Build history of the part. All positions in model axes, mm. Face numbers are marked on the shaded views. A direction names the side the tool comes from. Give positions to 0.01 mm unless a question says otherwise; leave off trailing zeros. Write each loop counter-clockwise with the first axis right and the second up, starting at its lowest first coordinate (ties: lowest second). Pieces come first, ordered by that corner, then holes. Notation, with made-up numbers: (4, 0) -> (13, 0) arc R18 ccw to (13, 18) -> close; hole circle Ø4 at (89.25, -21). An arc over 180 degrees is marked (long way). Put each result on its own line as item: value.
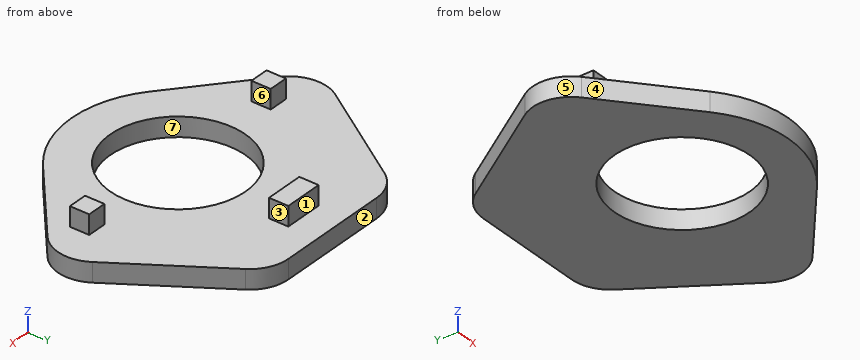
Autodesk Inventor part; units mm, degrees
ref_plane "YZ Plane" through (0, 0, 0) normal (1, 0, 0) x (0, 1, 0)
ref_plane "XZ Plane" through (0, 0, 0) normal (0, 1, 0) x (-1, 0, 0)
ref_plane "XY Plane" through (0, 0, 0) normal (0, 0, 1) x (1, 0, 0)
sketch "Sketch1" plane through (0, 0, 0) normal (0, 0, 1) x (1, 0, 0)
  circle A0 centre (0, 0) radius 7
  circle A1 centre (0, 0) radius 11
  line L0 (-31.215, 0) -> (-15, 0) construction
  line L1 (-11.7494, 0) -> (27.9854, 0) construction
  line L2 (7.0707, -8.4265) -> (18, 0.7443)
  line L3 (18, 0.7443) -> (8, 16)
  line L4 (8, 16) -> (0, 16)
  line L5 (0, -17.2006) -> (0, 31.2913) construction
  line L6 (-7.0707, -8.4265) -> (-18, 0.7443)
  line L7 (-18, 0.7443) -> (-8, 16)
  line L8 (-8, 16) -> (0, 16)
  dimension "d12" = 22
  dimension "d11" = 14
  dimension "d13" = 50
  dimension "d14" = 18
  dimension "d15" = 16
  dimension "d16" = 8
extrude "Extrusion1" add sketch "Sketch1" along normal blind 2
sketch "Sketch2" plane through (0, 0, 2) normal (0, 0, 1) x (1, 0, 0)
  arc A0 (-7.0707, -8.4265) -> (7.0707, -8.4265) centre (0, 0) ccw
  line L0 (7.0707, -8.4265) -> (18, 0.7443)
  line L1 (18, 0.7443) -> (8, 16)
  line L2 (8, 16) -> (-8, 16)
  line L3 (-8, 16) -> (-18, 0.7443)
  line L4 (-18, 0.7443) -> (-7.0707, -8.4265)
  circle A1 centre (0, 0) radius 7
  line L5 (11, -1) -> (13, -1)
  line L6 (13, -1) -> (13, 1)
  line L7 (13, 1) -> (11, 1)
  line L8 (11, 1) -> (11, -1)
  line L9 (11, -1) -> (13, 1) construction
  line L10 (13, -1) -> (11, 1) construction
  line L11 (-2, 13) -> (2, 13)
  line L12 (2, 13) -> (2, 11)
  line L13 (2, 11) -> (-2, 11)
  line L14 (-2, 11) -> (-2, 13)
  line L15 (-2, 13) -> (2, 11) construction
  line L16 (2, 13) -> (-2, 11) construction
  line L17 (0, 16) -> (0, -7) construction
  line L18 (-11, -1) -> (-13, -1)
  line L19 (-13, -1) -> (-13, 1)
  line L20 (-13, 1) -> (-11, 1)
  line L21 (-11, 1) -> (-11, -1)
  line L22 (-11, -1) -> (-13, 1) construction
  line L23 (-13, -1) -> (-11, 1) construction
  point P0 (12, 0)
  point P1 (0, 12)
  point P2 (12, 0)
  point P3 (0, 12)
  point P4 (0, 12)
  point P5 (-12, 0)
  point P6 (-12, 0)
  dimension "d18" = 2
  dimension "d19" = 2
  dimension "d20" = 4
  dimension "d21" = 2
  dimension "d22" = 12
  dimension "d23" = 12
extrude "Extrusion2" add sketch "Sketch2" along normal blind 2 contours L8 L7 L6 L5 | L11 L12 L13 L14 | L18 L19 L20 L21
fillet "Fillet1" radius 4 4 edges at (18, 0.7443, 1) (-18, 0.7443, 1) (-8, 16, 1) (8, 16, 1)
properties part number "lager opvulling voor lijm"
1) Tool access for the marked faces 1, 2 and 3: list every direction of +Z, -Z, +X, -X, +Y, -Y with a clear straight run to the whole face (end or side of a thin tool).
Filled sheet:
face 1: +Z, +X, -X, +Y
face 2: +Z, -Z, +X, -X, +Y
face 3: +Z, +X, +Y, -Y
2) Pin check, flat tips, straight feed: pin 1 (3 mm diameter, centred on x = 4.5, y = 1, fed in from -Z); pin 2 (1.5 mm diameter, centred on x = -5, y = 13, fed in from +Z); pin 3 (1.5 mm diameter, centred on x = 6.5, y = -4, fed in from -Z); pin 4 (1 mm diameter, centred on x = -12.5, z = 3, fed in from +Y). Stop position of each tip, or through.
Filled sheet:
pin 1: through
pin 2: z = 2
pin 3: z = 0
pin 4: y = 1
3) Slice it at B-B (y = -4.5). Write the cut outline in (x, z), plus the area to 3 significant figures.
Filled sheet:
outline: (-11.75, 0) -> (-5.36, 0) -> (-5.36, 2) -> (-11.75, 2) -> close; (5.36, 0) -> (11.75, 0) -> (11.75, 2) -> (5.36, 2) -> close
area: 25.6 mm2
4) Slice it at C-C (z = 2.45). Write the cut outline in (x, y), plus the area to 3 significant figures.
Filled sheet:
outline: (-13, -1) -> (-11, -1) -> (-11, 1) -> (-13, 1) -> close; (-2, 11) -> (2, 11) -> (2, 13) -> (-2, 13) -> close; (11, -1) -> (13, -1) -> (13, 1) -> (11, 1) -> close
area: 16.0 mm2
5) Pull direction Y, two halves, no side cores. Call the marked faces 4, 5, 6 and 7: released by +Y, released by -Y, zero draft, split by the parting line, or undercut.
Filled sheet:
face 4: released by -Y
face 5: split by the parting line
face 6: zero draft
face 7: undercut
6) Slice it at A-A (x = 0). Write the cut outline in (y, z), plus the area to 3 significant figures.
Filled sheet:
outline: (-11, 0) -> (-7, 0) -> (-7, 2) -> (-11, 2) -> close; (7, 0) -> (16, 0) -> (16, 2) -> (13, 2) -> (13, 4) -> (11, 4) -> (11, 2) -> (7, 2) -> close
area: 30.0 mm2
7) Wall check: L1, parallel to Y at x = 0, z = 0.65; L2, parallel to Z at x = 9.5, y = 11.25; L3, parallel to Y at x = -12, z = 2.35. Give the ranges that are in metal, low to high.
Filled sheet:
L1: -11 to -7, 7 to 16
L2: 0 to 2
L3: -1 to 1
8) Slice it at D-D (y = 12.5). Write the cut outline in (x, z).
Filled sheet:
outline: (-10.29, 0) -> (10.29, 0) -> (10.29, 2) -> (2, 2) -> (2, 4) -> (-2, 4) -> (-2, 2) -> (-10.29, 2) -> close
